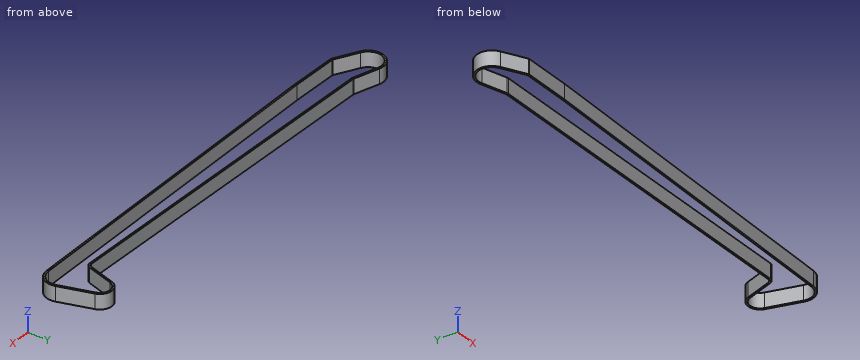
from build123d import *

# Parameters (mm, degrees)
EXTRUDE_1_DEPTH = 5
FILLET_1_R      = 0.3
FILLET_2_R      = 1.5


with BuildPart() as part:
    # 草图1 → 凸台-拉伸1 (new, symmetric)
    with BuildSketch(Plane.XY):
        with BuildLine():
            Line((141.619460126, 24.871545359), (148.401478886, 3.081820222))
            ThreePointArc((148.401478886, 3.081820222), (146.940254144, -6.024865973), (138.802378413, -10.365590543))
            Line((138.802378413, -10.365590543), (-95.482500904, -17.2))
            Line((-95.482500904, -17.2), (-127.791520657, -17.2))
            Line((-127.791520657, -17.2), (-143.257666119, -9.214201707))
            ThreePointArc((-143.257666119, -9.214201707), (-148.121840336, 3.867439534), (-135.557264597, 9.943701944))
            Line((-135.557264597, 9.943701944), (-119.199434765, 5.102771952))
            ThreePointArc((-119.199434765, 5.102771952), (-118.848420061, 5.025826388), (-118.49, 5))
            Line((-118.49, 5), (118.49, 5))
            ThreePointArc((118.49, 5), (119.978829003, 5.491670296), (120.882047608, 6.773289439))
            Line((120.882047608, 6.773289439), (126.364584034, 24.819660109))
            ThreePointArc((126.364584034, 24.819660109), (133.97285839, 30.479953843), (141.619460126, 24.871545359))
        make_face()
        with BuildLine():
            Line((-135.897793284, 8.793032481), (-119.539963452, 3.952102489))
            ThreePointArc((-119.539963452, 3.952102489), (-119.02046169, 3.838223055), (-118.49, 3.8))
            Line((-118.49, 3.8), (118.49, 3.8))
            ThreePointArc((118.49, 3.8), (120.693466924, 4.527672038), (122.030230461, 6.42446837))
            Line((122.030230461, 6.42446837), (127.512766886, 24.47083904))
            ThreePointArc((127.512766886, 24.47083904), (133.976939835, 29.279960784), (140.473676648, 24.514921996))
            Line((140.473676648, 24.514921996), (147.255695408, 2.725196859))
            ThreePointArc((147.255695408, 2.725196859), (145.963561282, -5.327678011), (138.767387661, -9.166100798))
            Line((138.767387661, -9.166100798), (-95.5, -16))
            Line((-95.5, -16), (-127.5, -16))
            Line((-127.5, -16), (-142.70711652, -8.147948858))
            ThreePointArc((-142.70711652, -8.147948858), (-147.008416189, 3.419905548), (-135.897793284, 8.793032481))
        make_face(mode=Mode.SUBTRACT)
    extrude(amount=EXTRUDE_1_DEPTH, both=True)

    # 圆角1
    fillet_1_edges = [part.edges().sort_by_distance(p)[0] for p in [
        (-127.5, -16, 0),
        (-95.5, -16, 0),
    ]]
    fillet(fillet_1_edges, radius=FILLET_1_R)

    # 圆角2
    fillet_2_edges = [part.edges().sort_by_distance(p)[0] for p in [
        (-95.482500904, -17.2, 0),
        (-127.791520657, -17.2, 0),
    ]]
    fillet(fillet_2_edges, radius=FILLET_2_R)


solid = part.part
Verification items for the finished model (mm, model axes). Give positions to 0.01 mm unless a question says otherwise; leave off trailing zeros. Order: outer loops, then holes, each group sorted by start corner. A loop starts at its lowest first (then second) coordinate and runs counter-clockwise, first axis right, second up. Notation, with made-up numbers: M 62.25,3 L 95.25,3 A18 cw 95.25,35 Z; hole C -28,-2 d4. An arc over 180 degrees is marked long. Use one line per item in the form item = value. Start each with the question number.
Q1. Section check B-B (y = 18). Enter the section's corners in (x, z).
Q2. Section check A-A (z = -1.5). Enter the section's corners in (x, y).
Q3. Scan lines: line 1 along Y through (x, z) = (-123.5, -3.5); line 2 along Y through (x, z) = (-118, -4); line 3 along X through (y, z) = (14, 0). Record each from-to range of solid material in increasing order. Write a range as [from, to].
Q4. Section check C-C (x = -60). Enter the section's corners in (y, z), then the cut area to 3 significant figures.
Q5. Go/stop test with flat-tipped pins: pin 1 Ø12 at (x, y) = (-117, -2.5) entering from +Z; pin 2 Ø3 at (x, z) = (87.5, 3) entering from -Y; pin 3 Ø6 at (x, z) = (-31, -1) entering from -Y; pin 4 Ø6 at (x, z) = (113, 3) entering from +Y. Record where each tip stops, or that it passes through.
Evaluation:
q1.outline = M 124.29,-5 L 125.55,-5 L 125.55,5 L 124.29,5 Z; M 142.5,-5 L 143.76,-5 L 143.76,5 L 142.5,5 Z
q2.outline = M -143.26,-9.21 L -128.12,-17.03 A1.5 ccw -127.43,-17.2 L -95.48,-17.2 L 138.8,-10.37 A10.37 ccw 148.4,3.08 L 141.62,24.87 A7.98 ccw 126.36,24.82 L 120.88,6.77 A2.5 cw 118.49,5 L -118.49,5 A2.5 cw -119.2,5.1 L -135.56,9.94 A10.37 ccw Z; hole M -142.71,-8.15 L -127.56,-15.97 A0.3 ccw -127.43,-16 L -95.5,-16 L 138.77,-9.17 A9.17 ccw 147.26,2.73 L 140.47,24.51 A6.78 ccw 127.51,24.47 L 122.03,6.42 A3.7 cw 118.49,3.8 L -118.49,3.8 A3.7 cw -119.54,3.95 L -135.9,8.79 A9.17 ccw Z
q3.line_1 = [-17.2, -16], [5.12, 6.38]
q3.line_2 = [-17.2, -16], [3.8, 5]
q3.line_3 = [123.08, 124.33], [143.75, 145]
q4.outline = M -16.16,-5 L -14.96,-5 L -14.96,5 L -16.16,5 Z; M 3.8,-5 L 5,-5 L 5,5 L 3.8,5 Z
q4.area = 24.0 mm2
q5.pin_1 = through
q5.pin_2 = -11.91
q5.pin_3 = -15.41
q5.pin_4 = 5
